Geometry: final body of the model. Coordinates: model frame, mm. A direction names the side the tool comes from. Give positions to 0.01 mm unless a question says otherwise; leave off trailing zeros. Loops run counter-clockwise (first coordinate to the right, second up) from the corner with the lowest first, then second, coordinate; pieces in that order, holes last.
1. First-contact query: P1, Ø1, axis at x = 3, y = 4, coming from the +Z side; P2, Ø4, axis at x = 1, z = -21, coming from the -Y side; P3, Ø2, axis at y = 3.5, z = -12.5, coming from the +X side; P4, Ø6, axis at y = 2.5, z = -28, coming from the -X side. Flat tips, straight axial feed; report the tip coordinate or a pass-through.
2. Access query for faces 1 (the face through (-3, 6, -29)), 2 (the face through (2.52, 1.9, -34.75)). Directions: +Z, -Z, +X, -X, +Y, -Y. A direction counts if a zero-diameter tool reaches every point of the face in a straight line with its end or side. Return the directions, or none.
3. Section A-A, the plane x = -0.5. Output: boundary loops of the cut face in (y, z).
4. Section C-C, the plane z = -40. Output: boundary loops of the cut face in (x, y).
5. Draft query along Y for faces 3 (the face through (-0.06, 7.63, -37.12)), 4 (the face through (0.1, -2.6, 2.7)), 5 (the face through (3, 2, -12)). Return one class per face: +Y half, -Y half, draft (parallel to the pull), parting line (faces both ways), or undercut.
6. Section D-D, the plane z = -13.5. Output: boundary loops of the cut face in (x, y).
7. Section B-B, the plane y = -1. Output: boundary loops of the cut face in (x, z).
8. Material intervals for line 1 along Z through (x, y) = (2, 4.75); line 2 along Z through (x, y) = (-1.25, 1); line 3 along Z through (x, y) = (-3, -0.5), sorted ascending.
from build123d import *

# Parameters (mm, degrees)
SKETCH_1_R          = 1.5
EXTRUDE_1_DEPTH     = 4
FILLET_1_R          = 2
FILLET_2_R          = 5
CUT_EXTRUDE_1_DEPTH = 3
FILLET_3_R          = 1


with BuildPart() as part:
    # 草图1 → 凸台-拉伸1 (new, symmetric)
    with BuildSketch(Plane(origin=(0, 0, 0), x_dir=(0, 0, -1), z_dir=(1, 0, 0))):
        with BuildLine():
            Line((2.651650429, -2.651650429), (5.303300859, 0))
            Line((5.303300859, 0), (34.696699141, 0))
            Line((34.696699141, 0), (37.348349571, -2.651650429))
            ThreePointArc((37.348349571, -2.651650429), (42.651650429, -2.651650429), (42.651650429, 2.651650429))
            Line((42.651650429, 2.651650429), (37.303300859, 8))
            Line((37.303300859, 8), (2.696699141, 8))
            Line((2.696699141, 8), (-2.651650429, 2.651650429))
            ThreePointArc((-2.651650429, 2.651650429), (-2.651650429, -2.651650429), (2.651650429, -2.651650429))
        make_face()
        Circle(SKETCH_1_R, mode=Mode.SUBTRACT)
        with Locations((40, 0)):
            Circle(SKETCH_1_R, mode=Mode.SUBTRACT)
    extrude(amount=EXTRUDE_1_DEPTH, both=True)

    # 圆角1
    fillet_1_edges = [part.edges().sort_by_distance(p)[0] for p in [
        (0, 0, -34.696699141),
        (0, 0, -5.303300859),
    ]]
    fillet(fillet_1_edges, radius=FILLET_1_R)

    # 圆角2
    fillet_2_edges = [part.edges().sort_by_distance(p)[0] for p in [
        (0, 8, -2.696699141),
        (0, 8, -37.303300859),
    ]]
    fillet(fillet_2_edges, radius=FILLET_2_R)

    # 草图2 → 切除-拉伸1 (cut)
    with BuildSketch(Plane(origin=(4, 0, 0), x_dir=(0, 0, -1), z_dir=(1, 0, 0))):
        with BuildLine():
            Line((18, 6), (18, 2))
            Line((18, 2), (6.131727984, 2))
            ThreePointArc((6.131727984, 2), (4.780909332, 1.765008496), (3.588806135, 1.087644486))
            ThreePointArc((3.588806135, 1.087644486), (2.659081759, 2.644198215), (1.107771013, 3.582644747))
            Line((1.107771013, 3.582644747), (2.646446609, 5.121320344))
            ThreePointArc((2.646446609, 5.121320344), (3.619716656, 5.771638598), (4.767766953, 6))
            Line((4.767766953, 6), (18, 6))
        make_face()
        with BuildLine():
            Line((22, 2), (22, 6))
            Line((22, 6), (35.232233047, 6))
            ThreePointArc((35.232233047, 6), (36.380283344, 5.771638598), (37.353553391, 5.121320344))
            Line((37.353553391, 5.121320344), (38.892228987, 3.582644747))
            ThreePointArc((38.892228987, 3.582644747), (37.340918241, 2.644198215), (36.411193865, 1.087644486))
            ThreePointArc((36.411193865, 1.087644486), (35.219090668, 1.765008496), (33.868272016, 2))
            Line((33.868272016, 2), (22, 2))
        make_face()
    cut_extrude_1 = extrude(amount=-CUT_EXTRUDE_1_DEPTH, mode=Mode.SUBTRACT)

    # 镜向1: 切除-拉伸1 across plane
    add(cut_extrude_1.mirror(Plane(origin=(0, 0, 0), x_dir=(0, 0, 1), z_dir=(1, 0, 0))), mode=Mode.SUBTRACT)

    # 圆角3
    fillet_3_edges = [part.edges().sort_by_distance(p)[0] for p in [
        (-2.5, 1.087644486, -36.411193865),
        (-2.5, 3.582644747, -38.892228987),
        (-2.5, 6, -22),
        (-2.5, 2, -22),
        (-2.5, 6, -18),
        (-2.5, 3.582644747, -1.107771013),
        (-2.5, 1.087644486, -3.588806135),
        (-2.5, 2, -18),
        (2.5, 1.087644486, -36.411193865),
        (2.5, 2, -22),
        (2.5, 6, -22),
        (2.5, 3.582644747, -38.892228987),
        (2.5, 6, -18),
        (2.5, 2, -18),
        (2.5, 1.087644486, -3.588806135),
        (2.5, 3.582644747, -1.107771013),
    ]]
    fillet(fillet_3_edges, radius=FILLET_3_R)


solid = part.part
Answers below:
1. P1: stops at z = 1.8
1. P2: stops at y = 0
1. P3: stops at x = 1
1. P4: stops at x = -4
2. face 1: -X
2. face 2: +X
3. outline: (-2.65, -37.35) arc R3.75 ccw to (2.65, -42.65) - (6.54, -38.77) arc R5 ccw to (8, -35.23) - (8, -4.77) arc R5 ccw to (6.54, -1.23) - (2.65, 2.65) arc R3.75 ccw to (-2.65, -2.65) - (-0.59, -4.72) arc R2 cw to (0, -6.13) - (0, -33.87) arc R2 cw to (-0.59, -35.28) - close; hole circle Ø3 at (0, -40); hole circle Ø3 at (0, 0)
4. outline: (-4, -3.75) - (4, -3.75) - (4, -1.5) - (-4, -1.5) - close; (-4, 1.5) - (4, 1.5) - (4, 5.3) - (-4, 5.3) - close
5. face 3: +Y half
5. face 4: parting line
5. face 5: undercut
6. outline: (-4, 0) - (4, 0) - (4, 2) - (1, 2) - (1, 6) - (4, 6) - (4, 8) - (-4, 8) - (-4, 6) - (-1, 6) - (-1, 2) - (-4, 2) - close
7. outline: (-4, -43.61) - (4, -43.61) - (4, -41.12) - (-4, -41.12) - close; (-4, -38.88) - (4, -38.88) - (4, -35.7) - (-4, -35.7) - close; (-4, -4.3) - (4, -4.3) - (4, -1.12) - (-4, -1.12) - close; (-4, 1.12) - (4, 1.12) - (4, 3.61) - (-4, 3.61) - close
8. line 1: z = -40.55 to -37.72, -22 to -18, -2.28 to 0.55
8. line 2: z = -43.61 to -41.12, -38.88 to -1.12, 1.12 to 3.61
8. line 3: z = -43.72 to -41.41, -38.59 to -35.19, -4.81 to -1.41, 1.41 to 3.72
